Input: dimensioned drawing with shaded views. Units: mm. Origin: part minimum x, y, z. Round coordinates to 2 decimals unless told otherwise and drop trailing zeros. Loops run counter-clockwise (first coordinate to the right, second up) from the corner with the lowest first, then second, coordinate; pieces in that order, holes last. Notation, with made-up numbers: M 77,-30.5 L 103,-30.5 A17 ccw 103,-17.5 Z; hole C -23.5,87 d3. An arc over 180 degrees is marked long. Use one line per item in the form item = value. Start each with the question number.
Q1. Section query B-B, the plane x = 50. Output: boundary loops of the cut face in (y, z), and give its area (3 significant figures).
Q2. Section query A-A, the plane z = 23. Output: boundary loops of the cut face in (x, y), and give its area (3 significant figures).
Q3. Section query C-C, the plane y = 9. Output: boundary loops of the cut face in (x, z).
Q4. Ray query, line 1 along X through (y, z) = (23, 23); line 2 along X through (y, z) = (31, 10.5) (1 decimal); line 3 along Y through (x, z) = (22, 17.5). Return the intervals inside material, ascending.
Q5. Mould query, pull axis X, two halves, no side actions, for the marked faces 1, 2, 3 and 4. Classes: pulls with the +X half, pulls with the -X half, needs draft (parallel to the pull), parting line crosses it, or undercut.
Q6. First-contact query: P1, Ø7, axis at x = 76, z = 23.5, coming from the -Y side; P2, Ø5.5, axis at x = 24, y = 31, coming from the -Z side. Flat tips, straight axial feed; report the tip coordinate or a pass-through.
Q7. Section query D-D, the plane z = 35.5. Output: boundary loops of the cut face in (x, y), and give its area (3 significant figures).
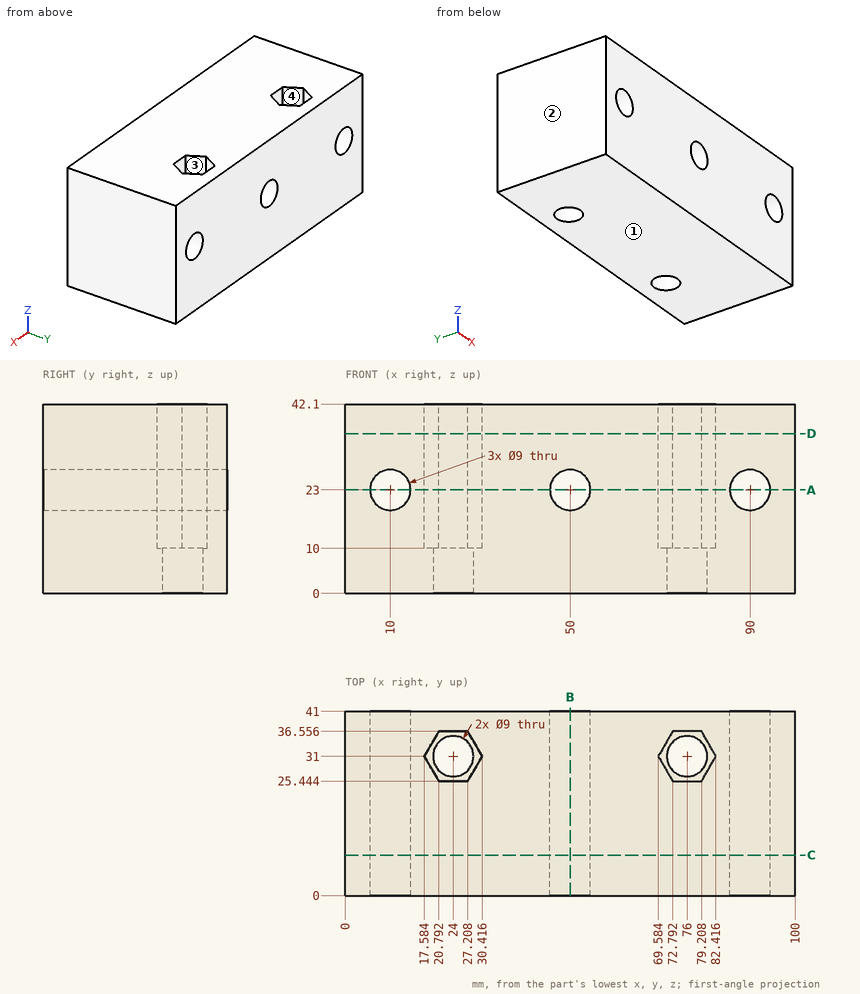
Results found:
q1.outline = M 0,0 L 41,0 L 41,18.5 L 0,18.5 Z; M 0,27.5 L 41,27.5 L 41,42.1 L 0,42.1 Z
q1.area = 1,360 mm²
q2.outline = M 0,0 L 5.5,0 L 5.5,41 L 0,41 Z; M 14.5,0 L 45.5,0 L 45.5,41 L 14.5,41 Z; M 54.5,0 L 85.5,0 L 85.5,41 L 54.5,41 Z; M 94.5,0 L 100,0 L 100,41 L 94.5,41 Z; hole M 17.58,31 L 20.79,25.44 L 27.21,25.44 L 30.42,31 L 27.21,36.56 L 20.79,36.56 Z; hole M 69.58,31 L 72.79,25.44 L 79.21,25.44 L 82.42,31 L 79.21,36.56 L 72.79,36.56 Z
q2.area = 2,780 mm²
q3.outline = M 0,0 L 100,0 L 100,42.1 L 0,42.1 Z; hole C 10,23 d9; hole C 50,23 d9; hole C 90,23 d9
q4.line_1 = 0 to 5.5, 14.5 to 45.5, 54.5 to 85.5, 94.5 to 100
q4.line_2 = 0 to 17.6, 30.4 to 69.6, 82.4 to 100
q4.line_3 = 0 to 25.44, 36.56 to 41
q5.face_1 = needs draft
q5.face_2 = pulls with the -X half
q5.face_3 = undercut
q5.face_4 = undercut
q6.P1 = 0
q6.P2 = through
q7.outline = M 0,0 L 100,0 L 100,41 L 0,41 Z; hole M 17.58,31 L 20.79,25.44 L 27.21,25.44 L 30.42,31 L 27.21,36.56 L 20.79,36.56 Z; hole M 69.58,31 L 72.79,25.44 L 79.21,25.44 L 82.42,31 L 79.21,36.56 L 72.79,36.56 Z
q7.area = 3,890 mm²
